Read the model definition and answer for the solid it produces. Units are mm, in the model's axes. A direction names the side the tool comes from. Round coordinates to 2 decimals unless told otherwise and drop trailing zeros. Write each loop counter-clockwise with the first axis right and the second up, starting at its lowest first coordinate (ties: lowest second). Pieces come first, ordered by that corner, then holes. Notation, with made-up numbers: (-2.75, 66) -> (8.25, 66) arc R10 ccw to (8.25, 76) -> close; hole circle Ø4 at (-36, 68). An arc over 180 degrees is marked (long way). Return JSON: item names as keys, results as strings.
from build123d import *

# Parameters (mm, degrees)
SKETCH1_W           = 25.4
SKETCH1_H           = 44.45
BOSS_EXTRUDE1_DEPTH = 3
FILLET1_R           = 3.175


with BuildPart() as part:
    # Sketch1 → Boss-Extrude1 (new, symmetric)
    with BuildSketch(Plane(origin=(0, 0, 0), x_dir=(1, 0, 0), z_dir=(0, 1, 0))):
        Rectangle(SKETCH1_W, SKETCH1_H)
        with BuildLine():
            Line((-7.85, -15.875), (-7.85, 15.875))
            ThreePointArc((-7.85, 15.875), (-6.35, 17.375), (-4.85, 15.875))
            Line((-4.85, 15.875), (-4.85, -15.875))
            ThreePointArc((-4.85, -15.875), (-6.35, -17.375), (-7.85, -15.875))
        make_face(mode=Mode.SUBTRACT)
        with BuildLine():
            Line((4.85, -15.875), (4.85, 15.875))
            ThreePointArc((4.85, 15.875), (6.35, 17.375), (7.85, 15.875))
            Line((7.85, 15.875), (7.85, -15.875))
            ThreePointArc((7.85, -15.875), (6.35, -17.375), (4.85, -15.875))
        make_face(mode=Mode.SUBTRACT)
    extrude(amount=BOSS_EXTRUDE1_DEPTH, both=True)

    # Fillet1
    fillet1_edges = [part.edges().sort_by_distance(p)[0] for p in [
        (-12.7, 0, -22.225),
        (12.7, 0, -22.225),
        (12.7, 0, 22.225),
        (-12.7, 0, 22.225),
    ]]
    fillet(fillet1_edges, radius=FILLET1_R)


solid = part.part
Item 1: Section B-B (x = 6.35) is taken. Give the vertices of the cut face in (y, z) (3 decimals).
Worked answers:
{"outline": "(-3, -22.225) -> (3, -22.225) -> (3, -17.375) -> (-3, -17.375) -> close; (-3, 17.375) -> (3, 17.375) -> (3, 22.225) -> (-3, 22.225) -> close"}
Item 2: A tool of negligible diameter and unlimited length cuts with its end or side. For faces 4 (the flat face through (0, 3, 0)), 5 (the flat face through (-4.85, 0, 0)), from which of +Z, -Z, +X, -X, +Y, -Y can it reach the whole face along a straight path? Write none if from no direction.
Worked answers:
{"face 4": "+Z, -Z, +X, -X, +Y", "face 5": "+Y, -Y"}
Item 3: For a pull along X with two mould halves and no side action, classify faces 1 (the flat face through (0, 0, 22.225)), 2 (the cylindrical face through (11.795, -0.042, -21.27)), 3 (the flat face through (4.85, 0, 0)) as released by +X, released by -X, zero draft, split by the parting line, or undercut.
Worked answers:
{"face 1": "zero draft", "face 2": "released by +X", "face 3": "undercut"}
Item 4: Section D-D (x = -6) is taken. Give the vertices of the cut face in (y, z) (3 decimals), then the cut area to 3 significant figures.
Worked answers:
{"outline": "(-3, -22.225) -> (3, -22.225) -> (3, -17.334) -> (-3, -17.334) -> close; (-3, 17.334) -> (3, 17.334) -> (3, 22.225) -> (-3, 22.225) -> close", "area": "58.7 mm2"}
Item 5: Straight lines are drawn through the part: L1, parallel to X at y = 2.15, z = -7; L2, parallel to X at y = -0.9, z = 17; L3, parallel to Z at x = -7.5, y = 1.7 (3 decimals). For each, find the intervals that lie inside material, in ascending order. Write a range as [from, to].
Worked answers:
{"L1": "x = [-12.7, -7.85], [-4.85, 4.85], [7.85, 12.7]", "L2": "x = [-12.7, -7.34], [-5.36, 5.36], [7.34, 12.7]", "L3": "z = [-22.225, -16.838], [16.838, 22.225]"}
Item 6: Section C-C (y = -0.8) is taken. Give the vertices of the cut face in (x, z) (3 decimals).
Worked answers:
{"outline": "(-12.7, -19.05) arc R3.175 ccw to (-9.525, -22.225) -> (9.525, -22.225) arc R3.175 ccw to (12.7, -19.05) -> (12.7, 19.05) arc R3.175 ccw to (9.525, 22.225) -> (-9.525, 22.225) arc R3.175 ccw to (-12.7, 19.05) -> close; hole (-7.85, -15.875) arc R1.5 ccw to (-4.85, -15.875) -> (-4.85, 15.875) arc R1.5 ccw to (-7.85, 15.875) -> close; hole (4.85, -15.875) arc R1.5 ccw to (7.85, -15.875) -> (7.85, 15.875) arc R1.5 ccw to (4.85, 15.875) -> close"}
Item 7: Section A-A (z = -9) is taken. Give the vertices of the cut face in (x, y).
Worked answers:
{"outline": "(-12.7, -3) -> (-7.85, -3) -> (-7.85, 3) -> (-12.7, 3) -> close; (-4.85, -3) -> (4.85, -3) -> (4.85, 3) -> (-4.85, 3) -> close; (7.85, -3) -> (12.7, -3) -> (12.7, 3) -> (7.85, 3) -> close"}
